Answer from the drawing. Dimensions are ordinates in mm from the lowest x, y and z of the part. Give positions to 0.01 mm unless a question says otherwise; leave off trailing zeros. Write each loop counter-clockwise with the first axis right and the second up, starting at its lowest first coordinate (ties: lowest second). Pieces come first, ordered by that corner, then holes.
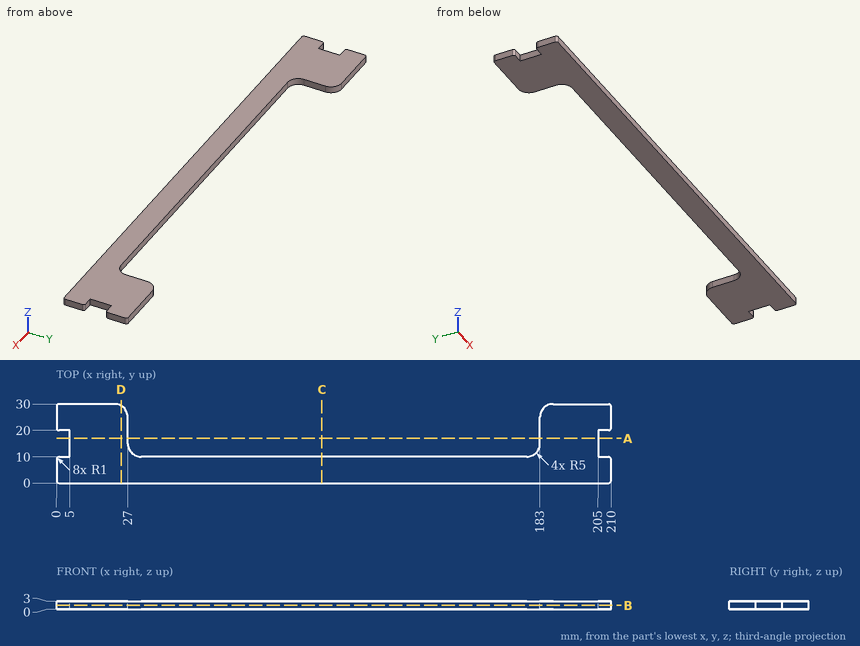
Item 1: Section D-D (x = 24.5) is taken. Write down the section's boundary in (y, z), and give its area (3 significant figures).
Result set:
outline: (0, 0) - (29.33, 0) - (29.33, 3) - (0, 3) - close
area: 88.0 mm2
Item 2: Each of these flat-tipped pins is pushed along its axis until it touches: pin 1 Ø0.9 at (y, z) = (18, 2) entering from +X; pin 2 Ø0.9 at (y, z) = (18.5, 1) entering from -X; pin 3 Ø1.5 at (x, z) = (139, 2) entering from +Y. Where does it stop, or does it pass through?
Result set:
pin 1: stops at x = 205
pin 2: stops at x = 5
pin 3: stops at y = 10
Item 3: Section A-A (y = 17) is taken. Write down the section's boundary in (x, z).
Result set:
outline: (5, 0) - (27, 0) - (27, 3) - (5, 3) - close; (183, 0) - (205, 0) - (205, 3) - (183, 3) - close
Item 4: Section C-C (x = 100.5) is taken. Write down the section's boundary in (y, z).
Result set:
outline: (0, 0) - (10, 0) - (10, 3) - (0, 3) - close
Item 5: Find the intervals of material crossed by line 1 along X through (y, z) = (21, 2.1); line 2 along X through (y, z) = (18.75, 0.95); line 3 along Y through (x, z) = (171.5, 0.8), in increasing order.
Result set:
line 1: x = 0 to 27, 183 to 210
line 2: x = 5 to 27, 183 to 205
line 3: y = 0 to 10
Item 6: Section B-B (z = 1.4) is taken. Write down the section's boundary in (x, y).
Result set:
outline: (0, 1) arc R1 ccw to (1, 0) - (209, 0) arc R1 ccw to (210, 1) - (210, 9) arc R1 ccw to (209, 10) - (205, 10) - (205, 20) - (209, 20) arc R1 ccw to (210, 21) - (210, 29) arc R1 ccw to (209, 30) - (188, 30) arc R5 ccw to (183, 25) - (183, 15) arc R5 cw to (178, 10) - (32, 10) arc R5 cw to (27, 15) - (27, 25) arc R5 ccw to (22, 30) - (1, 30) arc R1 ccw to (0, 29) - (0, 21) arc R1 ccw to (1, 20) - (5, 20) - (5, 10) - (1, 10) arc R1 ccw to (0, 9) - close
